Input: dimensioned drawing with shaded views. Units: mm. Origin: part minimum x, y, z. Coordinates: 2 decimals unless noted, no trailing zeros. Write each loop counter-clockwise with the first axis right and the second up, starting at its lowest first coordinate (ties: lowest second). Pieces come first, ordered by that corner, then holes. Notation, with made-up numbers: M 0.5,62.25 L 46.5,62.25 A13 cw 46.5,85.25 Z; hole C 60.5,1.5 d4. An arc over 180 degrees is marked long. Write each question's results on one line, items separated by ' | '. Start each with the question number.
1. Ray query, probe 1 along Y at (x, z) = (67.5, 1.25); probe 2 along Y at (x, z) = (6.35, 2.5); probe 3 along X at (y, z) = (6, 4.5) (1 decimal). Return the intervals inside material, ascending.
2. Section query A-A, the plane x = 53.5. Output: boundary loops of the cut face in (y, z), and give its area (3 significant figures).
3. Section query C-C, the plane x = 6.35. Output: boundary loops of the cut face in (y, z).
4. Section query B-B, the plane z = 4.25. Output: boundary loops of the cut face in (x, y), and give its area (3 significant figures).
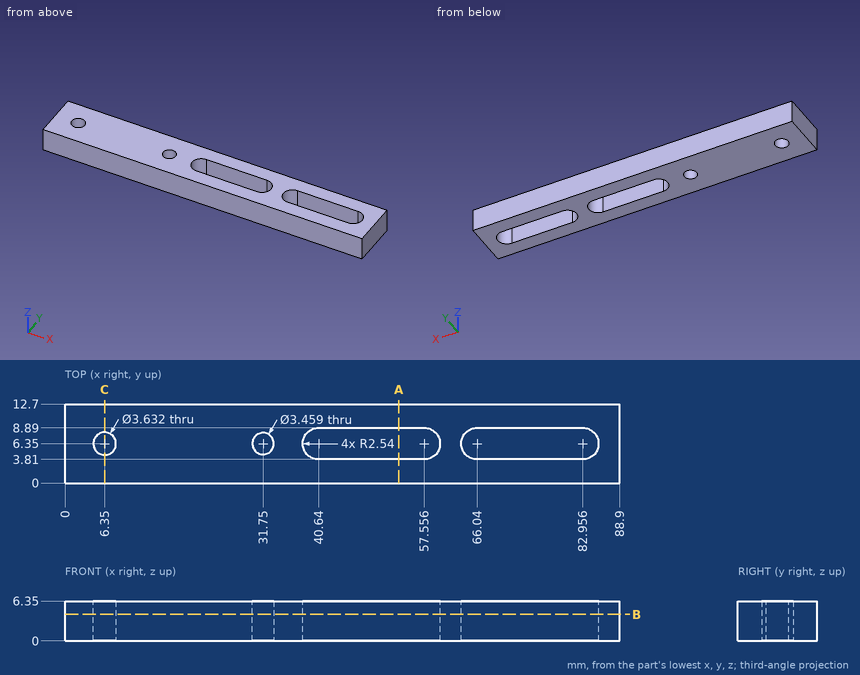
Answer:
1) probe 1: 0 to 3.81, 8.89 to 12.7 | probe 2: 0 to 4.53, 8.17 to 12.7 | probe 3: 0 to 4.6, 8.1 to 30.1, 33.4 to 38.1, 60.1 to 63.5, 85.5 to 88.9
2) outline: M 0,0 L 3.81,0 L 3.81,6.35 L 0,6.35 Z; M 8.89,0 L 12.7,0 L 12.7,6.35 L 8.89,6.35 Z | area: 48.4 mm^2
3) outline: M 0,0 L 4.53,0 L 4.53,6.35 L 0,6.35 Z; M 8.17,0 L 12.7,0 L 12.7,6.35 L 8.17,6.35 Z
4) outline: M 0,0 L 88.9,0 L 88.9,12.7 L 0,12.7 Z; hole C 6.35,6.35 d3.63; hole C 31.75,6.35 d3.46; hole M 40.64,3.81 L 57.56,3.81 A2.54 ccw 57.56,8.89 L 40.64,8.89 A2.54 ccw Z; hole M 66.04,3.81 L 82.96,3.81 A2.54 ccw 82.96,8.89 L 66.04,8.89 A2.54 ccw Z | area: 897 mm^2
